Verification items for this drawing (mm, ordinates from the low corner). Coordinates: 2 decimals unless noted, no trailing zeros. Order: outer loops, then holes, each group sorted by start corner. A loop starts at its lowest first (then second) coordinate and runs counter-clockwise, first axis right, second up.
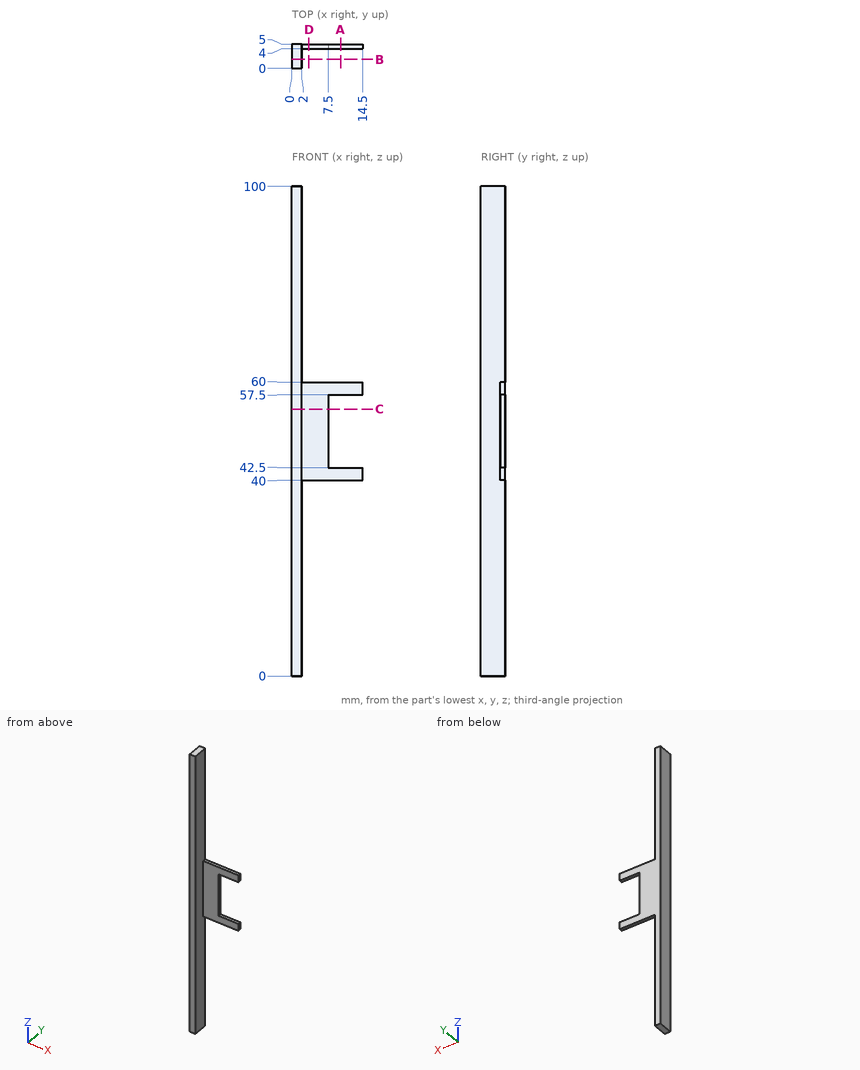
(1) Thickness scan on probe 1 along Z at (x, y) = (10.25, 4.1); probe 2 along X at (y, z) = (4.05, 64); probe 3 along Y at (x, z) = (14.25, 42). Record the ranges inside material, lowest first.
Filled in:
probe 1: z = 40 to 42.5, 57.5 to 60
probe 2: x = 0 to 2
probe 3: y = 4 to 5
(2) Cross-section at D-D (x = 3.5). Enter the section's corners in (y, z), and give its area (3 significant figures).
Filled in:
outline: (4, 40) - (5, 40) - (5, 60) - (4, 60) - close
area: 20.0 mm2
(3) Cross-section at B-B (y = 1.85). Enter the section's corners in (x, z).
Filled in:
outline: (0, 0) - (2, 0) - (2, 100) - (0, 100) - close
(4) Cross-section at C-C (z = 54.5). Enter the section's corners in (x, y), and give its area (3 significant figures).
Filled in:
outline: (0, 0) - (2, 0) - (2, 4) - (7.5, 4) - (7.5, 5) - (0, 5) - close
area: 15.5 mm2
(5) Cross-section at A-A (x = 10). Enter the section's corners in (y, z), and give its area (3 significant figures).
Filled in:
outline: (4, 40) - (5, 40) - (5, 42.5) - (4, 42.5) - close; (4, 57.5) - (5, 57.5) - (5, 60) - (4, 60) - close
area: 5.00 mm2
(6) Go/stop test with flat-tipped pins: P1, Ø3, axis at x = 4.5, z = 73, coming from the +Y side; P2, Ø0.5, axis at x = 7.5, y = 4.5, coming from the +Z side; P3, Ø1.5, axis at y = 2.5, z = 68.5, coming from the +X side; P4, Ø0.8, axis at x = 11.5, y = 4.5, coming from the -Z side. Record where each tip stops, or that it passes through.
Filled in:
P1: passes through
P2: stops at z = 60
P3: stops at x = 2
P4: stops at z = 40
